```python
from build123d import *

# Parameters (mm, degrees)
F0_W     = 70.66
F0_H     = 114.3
F1_DEPTH = 22
F0_H_2   = 12.7
F2_DEPTH = 7
F3_DEPTH = 82.55
F4_W     = 60.66
F4_H     = 74.3
F5_DEPTH = 40
F6_R     = 14.816073
F7_DEPTH = 20
F8_R     = 7.005396
F9_DEPTH = 20


with BuildPart() as f1:
    # F0 (on Top) → F1 (new body)
    with BuildSketch(Plane.XY):
        Rectangle(F0_W, F0_H)
    extrude(amount=-F1_DEPTH)

    # F0 (on Top) → F2 (join)
    with BuildSketch(Plane.XY):
        with Locations((0, -63.5)):
            Rectangle(F0_W, F0_H_2)
        with BuildLine():
            ThreePointArc((-2.921, -66.929), (-6.35, -63.5), (-2.921, -60.071))
            Line((-2.921, -60.071), (2.921, -60.071))
            ThreePointArc((2.921, -60.071), (5.345669, -61.075331), (6.35, -63.5))
            ThreePointArc((6.35, -63.5), (5.345669, -65.924669), (2.921, -66.929))
            Line((2.921, -66.929), (-2.921, -66.929))
        make_face(mode=Mode.SUBTRACT)
        with Locations((0, 63.5)):
            Rectangle(F0_W, F0_H_2)
        with BuildLine():
            ThreePointArc((2.921, 66.929), (5.345669, 65.924669), (6.35, 63.5))
            ThreePointArc((6.35, 63.5), (5.345669, 61.075331), (2.921, 60.071))
            Line((2.921, 60.071), (-2.921, 60.071))
            ThreePointArc((-2.921, 60.071), (-6.35, 63.5), (-2.921, 66.929))
            Line((-2.921, 66.929), (2.921, 66.929))
        make_face(mode=Mode.SUBTRACT)
    extrude(amount=-F2_DEPTH)

    # F0 (on Top) → F3 (join)
    with BuildSketch(Plane.XY):
        Polygon((-35.33, 69.85), (-36.83, 69.85), (-36.83, -69.85), (-35.33, -69.85), (-35.33, -57.15), (-35.33, 57.15), align=None)
        Polygon((36.83, 69.85), (35.33, 69.85), (35.33, 57.15), (35.33, -57.15), (35.33, -69.85), (36.83, -69.85), align=None)
    extrude(amount=-F3_DEPTH)

    # F4 (on face) → F5 (join)
    with BuildSketch(Plane(origin=(0, 0, -22), x_dir=(1, 0, 0), z_dir=(0, 0, -1))):
        Rectangle(F4_W, F4_H)
    extrude(amount=F5_DEPTH)

    # F6 (on face) → F7 (cut)
    with BuildSketch(Plane.XZ.offset(37.15)):
        with Locations((0, -42)):
            Circle(F6_R)
    extrude(amount=-F7_DEPTH, mode=Mode.SUBTRACT)

    # F8 (on face) → F9 (cut)
    with BuildSketch(Plane(origin=(0, 37.15, 0), x_dir=(-1, 0, 0), z_dir=(0, 1, 0))):
        with Locations((15.165, -32)):
            Circle(F8_R)
        with Locations((15.165, -52)):
            Circle(F8_R)
        with Locations((-15.165, -52)):
            Circle(F8_R)
        with Locations((-15.165, -32)):
            Circle(F8_R)
    extrude(amount=-F9_DEPTH, mode=Mode.SUBTRACT)


solid = f1.part
```
Input: part model. Units: mm. Frame: model coordinates. A direction names the side the tool comes from. Round coordinates to 2 decimals unless told otherwise and drop trailing zeros. Loops run counter-clockwise (first coordinate to the right, second up) from the corner with the lowest first, then second, coordinate; pieces in that order, holes last. Notation, with made-up numbers: (36, 52) - (53, 52) arc R7 cw to (53, 59) - close; hole circle Ø2 at (37, 21.25). An arc over 180 degrees is marked (long way). One line per item, written item: value. Start each with the question number.
(1) Section B-B, the plane z = -42. Return loops of the section in (x, y), plus the area to 3 significant figures.
(2) Section D-D, the plane z = -16. Return loops of the section in (x, y).
(3) Contact query for flat-ended pins moving along their axis: P1, Ø10, axis at x = -19.5, y = 26, coming from the +Z side; P2, Ø15.5, axis at x = -13.5, z = -49, coming from the +Y side; P3, Ø5, axis at x = 0, y = 8, coming from the -Z side; P4, Ø1.5, axis at x = 4, z = -15, coming from the +Y side. Output: stop coordinate, or through.
(4) Section C-C, the plane y = -24. Return loops of the section in (x, z), plus the area to 3 significant figures.
(5) Section A-A, the plane x = 0. Return loops of the section in (y, z).
(6) Draft query along Y for faces 6 (the cylindrical face through (-6.35, -63.58, -3.45)), 7 (the cylindrical face through (-18.398, 27.29, -58.215)), 8 (the flat face through (0, 66.929, -3)), 9 (the flat face through (-15, 17.15, -32)). Return one class per face: +Y half, -Y half, draft (parallel to the pull), parting line (faces both ways), or undercut.
(7) Ray query, line 1 (X direction, y = 1.5, z = -53); line 2 (Z direction, x = 0, y = -32); line 3 (Y direction, x = -21.5, z = -43.5). Return the intervals inside material, ascending. Write a range as [from, to].
(8) Access query for faces 1 (the flat face through (0, 57.15, -14)), 2 (the flat face through (15, 17.15, -52)), 3 (the flat face through (0, 60.071, -3)), 4 (the flat face through (30.33, 1, -42)), 5 (the flat face through (-7, -37.15, -28)). Directions: +Z, -Z, +X, -X, +Y, -Y. A direction counts if a zero-diameter tool reaches every point of the face in a straight line with its end or side. Return the directions, or none.
Results below:
1. outline: (-36.83, -69.85) - (-35.33, -69.85) - (-35.33, 69.85) - (-36.83, 69.85) - close; (-30.33, -37.15) - (-14.82, -37.15) - (-14.82, -17.15) - (14.82, -17.15) - (14.82, -37.15) - (30.33, -37.15) - (30.33, 37.15) - (-30.33, 37.15) - close; (35.33, -69.85) - (36.83, -69.85) - (36.83, 69.85) - (35.33, 69.85) - close
1. area: 4,330 mm^2
2. outline: (-36.83, -69.85) - (-35.33, -69.85) - (-35.33, -57.15) - (35.33, -57.15) - (35.33, -69.85) - (36.83, -69.85) - (36.83, 69.85) - (35.33, 69.85) - (35.33, 57.15) - (-35.33, 57.15) - (-35.33, 69.85) - (-36.83, 69.85) - close
3. P1: z = 0
3. P2: y = 37.15
3. P3: z = -62
3. P4: y = 57.15
4. outline: (-36.83, -82.55) - (-35.33, -82.55) - (-35.33, -22) - (-30.33, -22) - (-30.33, -62) - (30.33, -62) - (30.33, -22) - (35.33, -22) - (35.33, -82.55) - (36.83, -82.55) - (36.83, 0) - (-36.83, 0) - close; hole circle Ø29.63 at (0, -42)
4. area: 3,540 mm^2
5. outline: (-69.85, -7) - (-66.93, -7) - (-66.93, 0) - (-69.85, 0) - close; (-60.07, -7) - (-57.15, -7) - (-57.15, -22) - (-37.15, -22) - (-37.15, -27.18) - (-17.15, -27.18) - (-17.15, -56.82) - (-37.15, -56.82) - (-37.15, -62) - (37.15, -62) - (37.15, -22) - (57.15, -22) - (57.15, -7) - (60.07, -7) - (60.07, 0) - (-60.07, 0) - close; (66.93, -7) - (69.85, -7) - (69.85, 0) - (66.93, 0) - close
6. face 6: undercut
6. face 7: draft
6. face 8: undercut
6. face 9: +Y half
7. line 1: [-36.83, -35.33], [-30.33, 30.33], [35.33, 36.83]
7. line 2: [-62, -56.82], [-27.18, 0]
7. line 3: [-37.15, 37.15]
8. face 1: -Z, +Y
8. face 2: +Y
8. face 3: +Z, -Z
8. face 4: -Z, +Y, -Y
8. face 5: -Z, -Y
